Part model, mm, in its own coordinate system. A direction names the side the tool comes from. Coordinates: 2 decimals unless noted, no trailing zeros. Write each loop counter-clockwise with the first axis right and the second up, starting at its lowest first coordinate (ties: lowest second). Pieces come first, ordered by that corner, then holes. Notation, with made-up numbers: (57.25, -36.75) - (98.25, -36.75) arc R9 cw to (98.25, -24.75) - close; hole circle Ø11 at (86.5, 87.25). An arc over 180 degrees is marked (long way). Use a Markdown table: item, result.
```python
from build123d import *

# Parameters (mm, degrees)
ESQUISSE1_W        = 34
ESQUISSE1_H        = 15
ESQUISSE1_R        = 4
ESQUISSE1_R_2      = 2
BOSS_EXTRU_2_DEPTH = 10
ESQUISSE2_W        = 34
ESQUISSE2_H        = 18
ESQUISSE2_R        = 2
BOSS_EXTRU_3_DEPTH = 10
CHANFREIN1_SIZE    = 10
COQUE4_START       = 3
COQUE4_DEPTH       = 7
COQUE4_START_2     = 1
COQUE4_2_OUTLINE_W = 28
COQUE4_2_OUTLINE_H = 7
COQUE4_2_DEPTH     = 2
COQUE4_START_3     = 85.003902516
COQUE4_3_DEPTH     = 7
NERVURE3_REACH     = 97.863
ESQUISSE4_WALL_W   = 212.593996784
ESQUISSE4_WALL_H   = 3
CONG_1_R           = 10
CONG_2_R           = 1
CONG_3_R           = 4
NERVURE4_REACH     = 97.863
ESQUISSE6_WALL_W   = 210.930685054
ESQUISSE6_WALL_H   = 3


with BuildPart() as part:
    # Esquisse1 → Boss.-Extru.2 (new body)
    with BuildSketch(Plane.XY):
        with Locations((0, 74.503902516)):
            Rectangle(ESQUISSE1_W, ESQUISSE1_H)
        with Locations((-8, 74.003902516)):
            Circle(ESQUISSE1_R, mode=Mode.SUBTRACT)
        with Locations((8, 74.003902516)):
            Circle(ESQUISSE1_R_2, mode=Mode.SUBTRACT)
    extrude(amount=BOSS_EXTRU_2_DEPTH)

    # Esquisse2 → Boss.-Extru.3 (add)
    with BuildSketch(Plane(origin=(0, 82.003902516, 0), x_dir=(1, 0, 0), z_dir=(0, 1, 0))):
        with Locations((0, -1)):
            Rectangle(ESQUISSE2_W, ESQUISSE2_H)
        with Locations(Location((-8, 4, 0), (0, 0, 270))):
            Circle(ESQUISSE2_R, mode=Mode.SUBTRACT)
        with Locations(Location((8, 4, 0), (0, 0, 270))):
            Circle(ESQUISSE2_R, mode=Mode.SUBTRACT)
    extrude(amount=BOSS_EXTRU_3_DEPTH)

    # Chanfrein1
    chanfrein1_edges = [part.edges().sort_by_distance(p)[0] for p in [
        (0, 92.003902516, 10),
    ]]
    chamfer(chanfrein1_edges, length=CHANFREIN1_SIZE)

    # Coque4: read off the stored shape, not the designer's step
    # Coque4 outline → Coque4 (cut)
    with BuildSketch(Plane.XY.offset(COQUE4_START)):
        with BuildLine():
            Line((14, 70.003902516), (14, 92.003902516))
            Line((14, 92.003902516), (-14, 92.003902516))
            Line((-14, 92.003902516), (-14, 77.609453792))
            ThreePointArc((-14, 77.609453792), (-4.195080209, 79.87949486), (-2.255437353, 70.003902516))
            Line((-2.255437353, 70.003902516), (5, 70.003902516))
            ThreePointArc((5, 70.003902516), (8, 79.003902516), (11, 70.003902516))
            Line((11, 70.003902516), (14, 70.003902516))
        make_face()
        with BuildLine():
            Line((-14, 70.003902516), (-13.744562647, 70.003902516))
            ThreePointArc((-13.744562647, 70.003902516), (-13.875592344, 70.198982726), (-14, 70.398351241))
            Line((-14, 70.398351241), (-14, 70.003902516))
        make_face()
    extrude(amount=COQUE4_DEPTH, mode=Mode.SUBTRACT)

    # Coque4 2 outline → Coque4 2 (cut)
    with BuildSketch(Plane.XY.offset(COQUE4_START_2)):
        with Locations((0, 88.503902516)):
            Rectangle(COQUE4_2_OUTLINE_W, COQUE4_2_OUTLINE_H)
    extrude(amount=COQUE4_2_DEPTH, mode=Mode.SUBTRACT)

    # Coque4 3 outline → Coque4 3 (cut)
    with BuildSketch(Plane(origin=(0, 0, 0), x_dir=(1, 0, 0), z_dir=(0, 1, 0)).offset(COQUE4_START_3)):
        with BuildLine():
            Line((14, 5), (12.898979486, 5))
            ThreePointArc((12.898979486, 5), (11.872983347, 0.83772234), (8, -1))
            Line((8, -1), (14, -1))
            Line((14, -1), (14, 5))
        make_face()
        with BuildLine():
            Line((-14, -1), (-8, -1))
            ThreePointArc((-8, -1), (-11.872983346, 0.83772234), (-12.898979485, 5))
            Line((-12.898979485, 5), (-14, 5))
            Line((-14, 5), (-14, -1))
        make_face()
        with BuildLine():
            Line((-8, -1), (8, -1))
            ThreePointArc((8, -1), (4.127016654, 0.83772234), (3.101020515, 5))
            Line((3.101020515, 5), (-3.101020514, 5))
            ThreePointArc((-3.101020514, 5), (-4.127016653, 0.83772234), (-8, -1))
        make_face()
    extrude(amount=COQUE4_3_DEPTH, mode=Mode.SUBTRACT)

    # Esquisse4 wall → Nervure3 (add, up to next)
    with BuildSketch(Plane(origin=(8, 84.003902516, 5), x_dir=(0, 0.847998304005, -0.529998940003), z_dir=(0, -0.529998940003, -0.847998304005)), mode=Mode.PRIVATE) as nervure3_sk1:
        Rectangle(ESQUISSE4_WALL_W, ESQUISSE4_WALL_H)
    nervure3_tool1 = extrude(nervure3_sk1.sketch, amount=NERVURE3_REACH, mode=Mode.PRIVATE) - part.part
    add(nervure3_tool1.solids().sort_by_distance((8, 84.003902516, 5))[0])

    # Congé1
    cong_1_edges = [part.edges().sort_by_distance(p)[0] for p in [
        (-17, 67.003902516, 5),
    ]]
    fillet(cong_1_edges, radius=CONG_1_R)

    # Congé2
    cong_2_edges = [part.edges().sort_by_distance(p)[0] for p in [
        (14, 70.003902516, 6.5),
    ]]
    fillet(cong_2_edges, radius=CONG_2_R)

    # Congé3
    cong_3_edges = [part.edges().sort_by_distance(p)[0] for p in [
        (17, 67.003902516, 5),
    ]]
    fillet(cong_3_edges, radius=CONG_3_R)

    # Esquisse6 wall → Nervure4 (add, up to next)
    with BuildSketch(Plane(origin=(-8, 85.003902516, 5), x_dir=(0, -0.813733471207, 0.581238193719), z_dir=(0, 0.581238193719, 0.813733471207)), mode=Mode.PRIVATE) as nervure4_sk1:
        Rectangle(ESQUISSE6_WALL_W, ESQUISSE6_WALL_H)
    nervure4_tool1 = extrude(nervure4_sk1.sketch, amount=-NERVURE4_REACH, mode=Mode.PRIVATE) - part.part
    add(nervure4_tool1.solids().sort_by_distance((-8, 85.003902516, 5))[0])


solid = part.part
```
Item 1: Band-saw the part on B-B, the plane x = 4. Give the cut face in (y, z), then the cut area to 3 significant figures.
From the geometry:
| item | result |
|---|---|
| outline | (67, 0) - (82, 0) - (82, -8) - (92, -8) - (92, -1) - (85, -1) - (85, 3) - (77, 3) - (77, 10) - (71, 10) - (71, 3) - (70, 3) - (70, 10) - (67, 10) - close |
| area | 190 mm^2 |
Item 2: Band-saw the part on C-C, the plane y = 84. Give the cut face in (x, z).
From the geometry:
| item | result |
|---|---|
| outline | (-17, -8) - (17, -8) - (17, 8) - (14, 8) - (14, 3) - (9.5, 3) - (9.5, 5) - (6.5, 5) - (6.5, 3) - (-6.5, 3) - (-6.5, 5.72) - (-9.5, 5.72) - (-9.5, 3) - (-14, 3) - (-14, 8) - (-17, 8) - close; hole circle Ø4 at (-8, -4); hole circle Ø4 at (8, -4) |
Item 3: Band-saw the part on D-D, the plane z = 3.75. Give the cut face in (x, y).
From the geometry:
| item | result |
|---|---|
| outline | (-17, 77) arc R10 ccw to (-7, 67) - (13, 67) arc R4 ccw to (17, 71) - (17, 88.25) - (14, 88.25) - (14, 71) arc R1 cw to (13, 70) - (11, 70) arc R5 ccw to (9.5, 78.77) - (9.5, 86) - (6.5, 86) - (6.5, 78.77) arc R5 ccw to (5, 70) - (-2.26, 70) arc R7 ccw to (-6.5, 80.84) - (-6.5, 86.75) - (-9.5, 86.75) - (-9.5, 80.84) arc R7 ccw to (-14, 77.61) - (-14, 88.25) - (-17, 88.25) - close; hole (-14, 70) - (-13.74, 70) arc R7 cw to (-14, 70.4) - close; hole circle Ø8 at (-8, 74); hole circle Ø4 at (8, 74) |
Item 4: Which spindle directions (+Z, -Z, +X, -X, +Y, -Y) get a long thin tool onto all of the face, cutting with end or side? Do faces 1 (the face through (6.5, 83, 4)), 2 (the face through (-17, 84, 1)). Say none if no direction does.
From the geometry:
| item | result |
|---|---|
| face 1 | +Z, +Y |
| face 2 | +Z, -Z, -X, +Y, -Y |
Item 5: Drill centre lines: probe 1 along X at (y, z) = (82.25, -3.25); probe 2 along X at (y, z) = (77, 4.25); probe 3 along Z at (x, y) = (1, 84.5). Where is each one in solid material? Low to high.
From the geometry:
| item | result |
|---|---|
| probe 1 | -17 to -9.85, -6.15 to 6.15, 9.85 to 17 |
| probe 2 | -17 to -10.65, -5.35 to -1.67, 4 to 12, 14 to 17 |
| probe 3 | -8 to 3 |
Item 6: Band-saw the part on A-A, the plane z = -4. Give the cut face in (x, y), then the cut area to 3 significant figures.
From the geometry:
| item | result |
|---|---|
| outline | (-17, 82) - (-10, 82) - (-10, 92) - (-13, 92) - (-13, 85) - (-14, 85) - (-14, 92) - (-17, 92) - close; (-6, 82) - (6, 82) - (6, 92) - (3, 92) - (3, 85) - (-3, 85) - (-3, 92) - (-6, 92) - close; (10, 82) - (17, 82) - (17, 92) - (14, 92) - (14, 85) - (13, 85) - (13, 92) - (10, 92) - close |
| area | 204 mm^2 |
Item 7: Drop flat-ended pins along their axis: P1, Ø2, axis at x = 12.5, z = 8, coming from the +Y side; P2, Ø1, axis at x = 1.5, y = 83, coming from the +Z side; P3, Ø1.2, axis at x = -13, y = 89, coming from the +Z side. Give the stop position or say it passes through.
From the geometry:
| item | result |
|---|---|
| P1 | y = 77.57 |
| P2 | z = 3 |
| P3 | z = -1.63 |
